Part model, mm, in its own coordinate system. A direction names the side the tool comes from. Coordinates: 2 decimals unless noted, no trailing zeros. Order: outer loops, then holes, each group sorted by start corner. A loop starts at its lowest first (then second) coordinate and runs counter-clockwise, first axis right, second up.
```python
from build123d import *

# Parameters (mm, degrees)
F4_W = 99.84846
F4_H = 2.5


with BuildPart() as f3:
    # F3: sweep along a path in F2
    with BuildLine(Plane.YZ) as f3_path:
        Line((0, 60), (79.139297, 60))
    # F0 (on Front) → F3 (sweep)
    with BuildSketch(Plane.XZ):
        with BuildLine():
            Line((-84.816337, 27.746068), (-87, 0))
            Line((-87, 0), (-84.49227, 0))
            Line((-84.49227, 0), (-82.324044, 27.549921))
            ThreePointArc((-82.324044, 27.549921), (-71.985255, 48.865482), (-49.92423, 57.5))
            Line((-49.92423, 57.5), (0, 57.5))
            Line((0, 57.5), (49.92423, 57.5))
            ThreePointArc((49.92423, 57.5), (71.985255, 48.865482), (82.324044, 27.549921))
            Line((82.324044, 27.549921), (84.49227, 0))
            Line((84.49227, 0), (87, 0))
            Line((87, 0), (84.816337, 27.746068))
            ThreePointArc((84.816337, 27.746068), (73.682256, 50.701288), (49.92423, 60))
            Line((49.92423, 60), (0, 60))
            Line((0, 60), (-49.92423, 60))
            ThreePointArc((-49.92423, 60), (-73.682256, 50.701288), (-84.816337, 27.746068))
        make_face()
    sweep(path=f3_path.line)

    # F5: sweep along a path in F2
    with BuildLine(Plane.YZ) as f5_path:
        ThreePointArc((79.139297, 60), (85.862965, 57.402181), (89.093259, 50.958458))
        Line((89.093259, 50.958458), (94, 0))
    # F4 (on face) → F5 (sweep)
    with BuildSketch(Plane(origin=(0, 79.139297, 0), x_dir=(-1, 0, 0), z_dir=(0, 1, 0))):
        with Locations((0, 58.75)):
            Rectangle(F4_W, F4_H)
    sweep(path=f5_path.line)


solid = f3.part
```
(1) Probe line 1 (Z direction, x = -20.5, y = 39.5); line 2 (X direction, y = 17, z = 23); line 3 (X direction, y = 65, z = 7.5). List the from-to ranges inside material, lowest first.
(2) Slice it at C-C, the plane y = 44. Give the cut face in (x, z).
(3) Drop flat-ended pins along their axis: pin 1 (8 mm diameter, centred on x = -43, z = 11.5, fed in from -Y); pin 2 (7.5 mm diameter, centred on y = 85.5, z = 32, fed in from +X); pin 3 (3 mm diameter, centred on x = 86.5, y = 44, fed in from -Z); pin 4 (18.5 mm diameter, centred on x = 60.5, z = 39, fed in from +Y). Give the stop position or say it passes through.
(4) Slice it at B-B, the plane x = 43. Give the cut face in (y, z).
(5) Tool access for faces 1 (the face through (-73.9, 40.1, 50.5)), 2 (the face through (-1, 40, 57.5)), 3 (the face through (71.735, 40.124, 49.095)): list every direction of +Z, -Z, +X, -X, +Y, -Y with a clear straight run to the whole face (end or side of a thin tool).
(6) Slice it at D-D, the plane z = 34. Give the cut face in (x, y), then the cut area to 3 significant figures.
(7) Pull direction X, two halves, no side cores. Call faces 4 (the face through (85.923, 40.124, 13.679)), 5 (the face through (-83.423, 40.124, 13.582)), 6 (the face through (0, 0, 59)): +X half, -X half, draft (parallel to the pull), parting line (faces both ways), or undercut.
(8) Slice it at A-A, the plane z = 20.5. Give the cut face in (x, y), then the cut area to 3 significant figures.
Here are the results:
1. line 1: z = 57.5 to 60
1. line 2: x = -85.19 to -82.68, 82.68 to 85.19
1. line 3: x = -86.41 to -83.9, 83.9 to 86.41
2. outline: (-87, 0) - (-84.49, 0) - (-82.32, 27.55) arc R32.5 cw to (-49.92, 57.5) - (49.92, 57.5) arc R32.5 cw to (82.32, 27.55) - (84.49, 0) - (87, 0) - (84.82, 27.75) arc R35 ccw to (49.92, 60) - (-49.92, 60) arc R35 ccw to (-84.82, 27.75) - close
3. pin 1: stops at y = 90
3. pin 2: stops at x = 49.92
3. pin 3: stops at z = 0
3. pin 4: passes through
4. outline: (0, 57.5) - (79.14, 57.5) arc R7.5 cw to (86.6, 50.72) - (91.51, -0.24) - (94, 0) - (89.09, 50.96) arc R10 ccw to (79.14, 60) - (0, 60) - close
5. face 1: +Z, -X, +Y, -Y
5. face 2: -Z, -Y
5. face 3: -Z, +Y, -Y
6. outline: (-83.75, 0) - (-81.15, 0) - (-81.15, 79.14) - (-83.75, 79.14) - close; (-49.92, 88.21) - (49.92, 88.21) - (49.92, 90.73) - (-49.92, 90.73) - close; (81.15, 0) - (83.75, 0) - (83.75, 79.14) - (81.15, 79.14) - close
6. area: 661 mm2
7. face 4: +X half
7. face 5: undercut
7. face 6: draft
8. outline: (-85.39, 0) - (-82.88, 0) - (-82.88, 79.14) - (-85.39, 79.14) - close; (-49.92, 89.51) - (49.92, 89.51) - (49.92, 92.03) - (-49.92, 92.03) - close; (82.88, 0) - (85.39, 0) - (85.39, 79.14) - (82.88, 79.14) - close
8. area: 648 mm2
